The model under review builds one solid part; all positions refer to its coordinate system, in mm. Face numbers are marked on the shaded views. Round coordinates to 2 decimals unless told otherwise and drop trailing zeros. Write item = value, one per line. Start each with the question number.
Item 1: Take a section at A-A, the plane y = 15. Give the number of separate pieces and of enclosed holes in the cut face, plus the area to 3 significant figures.
Item 2: The part is to be moulded in two halves that separate along Z. For the marked faces 1, 2 and 3, say which applies: +Z half, -Z half, draft (parallel to the pull), parting line (faces both ways), or undercut.
Item 3: For pin 1 Ø1.1 at (x, z) = (87, 23.5) entering from +Y; pin 2 Ø5 at (x, z) = (15, 81.13) entering from +Y; pin 3 Ø6 at (y, z) = (8.5, 51) entering from +X, all flat-tipped, find the tip position at first contact; note any pin that passes through.
Item 4: To check wall thickness, follow line 1 along X through (y, z) = (17.5, 17); line 2 along X through (y, z) = (18.75, 62.5); line 3 along X through (y, z) = (3.25, 5). State the ranges of each line that lie inside material, in increasing order.
from build123d import *

# Parameters (mm, degrees)
SKETCH3_R           = 1.85
CUT_EXTRUDE1_DEPTH  = 155.06371723
SKETCH4_R           = 3.85
SKETCH4_R_2         = 1.85
BOSS_EXTRUDE1_DEPTH = 10
SKETCH_2_R          = 3.85
SKETCH_2_R_2        = 1.85
EXTRUDE_1_DEPTH     = 10


with BuildPart() as part:
    # Sketch1 → Loft1 section 0
    with BuildSketch(Plane(origin=(0, 0, 0), x_dir=(1, 0, 0), z_dir=(0, 1, 0))):
        with BuildLine():
            Line((0, 0), (127.35007717, 0))
            Line((127.35007717, 0), (127.35007717, -86.125413014))
            Line((127.35007717, -86.125413014), (0, -86.125413014))
            Line((0, -86.125413014), (0, 0))
        make_face()
    # Sketch2 → Loft1 section 1
    with BuildSketch(Plane(origin=(0, 10, 0), x_dir=(1, 0, 0), z_dir=(0, 1, 0))):
        with BuildLine():
            Line((10, -10), (10, -76.125413014))
            Line((10, -76.125413014), (117.35007717, -76.125413014))
            Line((117.35007717, -76.125413014), (117.35007717, -10))
            Line((117.35007717, -10), (10, -10))
        make_face()
    loft()

    # Sketch3 → Cut-Extrude1 (cut, through all)
    with BuildSketch(Plane.XZ):
        with Locations(Location((5, 15, 0), (0, 0, 270))):
            Circle(SKETCH3_R)
        with Locations(Location((5, 71.125413014, 0), (0, 0, 180))):
            Circle(SKETCH3_R)
        with Locations(Location((122.35007717, 71.125413014, 0), (0, 0, 270))):
            Circle(SKETCH3_R)
        with Locations((122.35007717, 15)):
            Circle(SKETCH3_R)
        with Locations(Location((15, 5, 0), (0, 0, 270))):
            Circle(SKETCH3_R)
        with Locations(Location((15, 81.125413014, 0), (0, 0, 270))):
            Circle(SKETCH3_R)
        with Locations(Location((112.35007717, 81.125413014, 0), (0, 0, 90))):
            Circle(SKETCH3_R)
        with Locations(Location((112.35007717, 5, 0), (0, 0, 270))):
            Circle(SKETCH3_R)
    extrude(amount=-CUT_EXTRUDE1_DEPTH, mode=Mode.SUBTRACT)

    # Sketch4 → Boss-Extrude1 (add)
    # profile 1 of 4: a face of its own
    with BuildSketch(Plane(origin=(0, 10, 0), x_dir=(1, 0, 0), z_dir=(0, 1, 0))):
        with Locations(Location((110.35007717, -69.125413014, 0), (0, 0, 270))):
            Circle(SKETCH4_R)
        with Locations(Location((110.35007717, -69.125413014, 0), (0, 0, 270))):
            Circle(SKETCH4_R_2, mode=Mode.SUBTRACT)
    # profile 2 of 4: a face of its own
    with BuildSketch(Plane(origin=(0, 10, 0), x_dir=(1, 0, 0), z_dir=(0, 1, 0))):
        with Locations(Location((110.35007717, -17, 0), (0, 0, 90))):
            Circle(SKETCH4_R)
        with Locations(Location((110.35007717, -17, 0), (0, 0, 90))):
            Circle(SKETCH4_R_2, mode=Mode.SUBTRACT)
    # profile 3 of 4: a face of its own
    with BuildSketch(Plane(origin=(0, 10, 0), x_dir=(1, 0, 0), z_dir=(0, 1, 0))):
        with Locations(Location((17, -17, 0), (0, 0, 270))):
            Circle(SKETCH4_R)
        with Locations(Location((17, -17, 0), (0, 0, 270))):
            Circle(SKETCH4_R_2, mode=Mode.SUBTRACT)
    # profile 4 of 4: a face of its own
    with BuildSketch(Plane(origin=(0, 10, 0), x_dir=(1, 0, 0), z_dir=(0, 1, 0))):
        with Locations(Location((17, -69.125413014, 0), (0, 0, 90))):
            Circle(SKETCH4_R)
        with Locations(Location((17, -69.125413014, 0), (0, 0, 90))):
            Circle(SKETCH4_R_2, mode=Mode.SUBTRACT)
    extrude(amount=BOSS_EXTRUDE1_DEPTH)

    # Эскиз2 → Бобышка-Вытянуть1 (add)
    # profile 1 of 4: a face of its own
    with BuildSketch(Plane(origin=(0, 10, 0), x_dir=(1, 0, 0), z_dir=(0, 1, 0))):
        with Locations(Location((87.35007717, -23.062706507, 0), (0, 0, 270))):
            Circle(SKETCH_2_R)
        with Locations(Location((87.35007717, -23.062706507, 0), (0, 0, 270))):
            Circle(SKETCH_2_R_2, mode=Mode.SUBTRACT)
    # profile 2 of 4: a face of its own
    with BuildSketch(Plane(origin=(0, 10, 0), x_dir=(1, 0, 0), z_dir=(0, 1, 0))):
        with Locations(Location((47.35007717, -23.062706507, 0), (0, 0, 270))):
            Circle(SKETCH_2_R)
        with Locations(Location((47.35007717, -23.062706507, 0), (0, 0, 270))):
            Circle(SKETCH_2_R_2, mode=Mode.SUBTRACT)
    # profile 3 of 4: a face of its own
    with BuildSketch(Plane(origin=(0, 10, 0), x_dir=(1, 0, 0), z_dir=(0, 1, 0))):
        with Locations(Location((47.35007717, -63.062706507, 0), (0, 0, 270))):
            Circle(SKETCH_2_R)
        with Locations(Location((47.35007717, -63.062706507, 0), (0, 0, 270))):
            Circle(SKETCH_2_R_2, mode=Mode.SUBTRACT)
    # profile 4 of 4: a face of its own
    with BuildSketch(Plane(origin=(0, 10, 0), x_dir=(1, 0, 0), z_dir=(0, 1, 0))):
        with Locations(Location((87.35007717, -63.062706507, 0), (0, 0, 270))):
            Circle(SKETCH_2_R)
        with Locations(Location((87.35007717, -63.062706507, 0), (0, 0, 270))):
            Circle(SKETCH_2_R_2, mode=Mode.SUBTRACT)
    extrude(amount=EXTRUDE_1_DEPTH)


solid = part.part
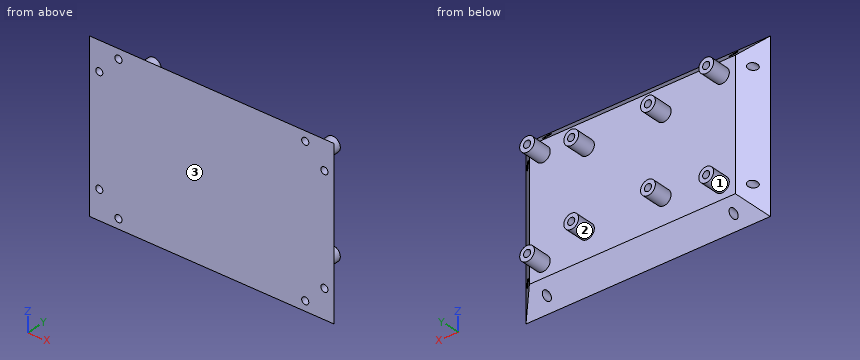
Response values:
q1.separate_pieces = 8
q1.enclosed_holes = 8
q1.area = 287 mm2
q2.face_1 = undercut
q2.face_2 = undercut
q2.face_3 = draft
q3.pin_1 = 10
q3.pin_2 = 7.5
q3.pin_3 = 121.85
q4.line_1 = 13.15 to 15.15, 18.85 to 20.85, 106.5 to 108.5, 112.2 to 114.2
q4.line_2 = 43.54 to 45.59, 49.11 to 51.16, 83.54 to 85.59, 89.11 to 91.16
q4.line_3 = 3.25 to 13.15, 16.85 to 110.5, 114.2 to 124.1
